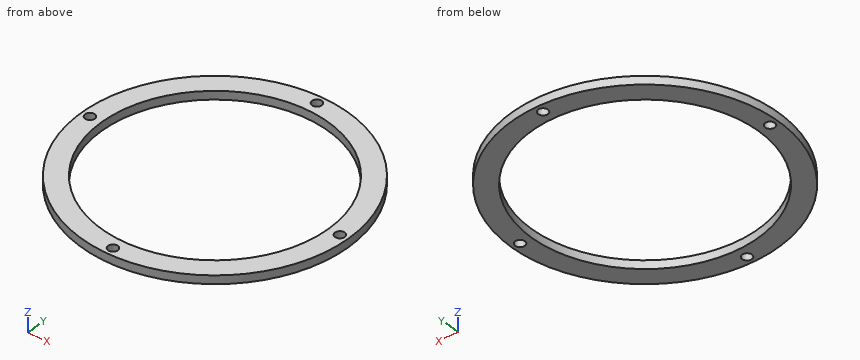
Autodesk Inventor part; units mm, degrees
ref_plane "YZ Plane" through (0, 0, 0) normal (1, 0, 0) x (0, 1, 0)
ref_plane "XZ Plane" through (0, 0, 0) normal (0, 1, 0) x (-1, 0, 0)
ref_plane "XY Plane" through (0, 0, 0) normal (0, 0, 1) x (1, 0, 0)
sketch "Sketch1" plane through (0, 0, 0) normal (0, 0, 1) x (1, 0, 0)
  circle A0 centre (0, 0) radius 48
  circle A1 centre (0, 0) radius 40.75
  line L0 (0, 0) -> (0, 45)
  circle A2 centre (0, 45) radius 1.75
  circle A3 centre (-45, 0) radius 1.75
  circle A4 centre (0, -45) radius 1.75
  circle A5 centre (45, 0) radius 1.75
  dimension "d0" = 96
  dimension "d1" = 81.5
  dimension "d2" = 45
  dimension "d3" = 3.5
  dimension "d6" = 360
extrude "Extrusion1" add sketch "Sketch1" along normal blind 3
properties part number "arm_0_bottom_top_lock"
Geometry check sheet. Reference: the model listing, model coordinates, mm. Give positions to 0.01 mm unless a question says otherwise; leave off trailing zeros. Order: outer loops, then holes, each group sorted by start corner. A loop starts at its lowest first (then second) coordinate and runs counter-clockwise, first axis right, second up.
1) Cross-section at C-C (y = -10). Record the boundary of the cut face in (x, z), then the cut area to 3 significant figures.
Results are:
outline: (-46.95, 0) - (-39.5, 0) - (-39.5, 3) - (-46.95, 3) - close; (39.5, 0) - (46.95, 0) - (46.95, 3) - (39.5, 3) - close
area: 44.7 mm2
2) Cross-section at A-A (y = 0). Record the boundary of the cut face in (x, z), then the cut area to 3 significant figures.
Results are:
outline: (-48, 0) - (-46.75, 0) - (-46.75, 3) - (-48, 3) - close; (-43.25, 0) - (-40.75, 0) - (-40.75, 3) - (-43.25, 3) - close; (40.75, 0) - (43.25, 0) - (43.25, 3) - (40.75, 3) - close; (46.75, 0) - (48, 0) - (48, 3) - (46.75, 3) - close
area: 22.5 mm2
3) Cross-section at D-D (x = -16). Record the boundary of the cut face in (y, z).
Results are:
outline: (-45.25, 0) - (-37.48, 0) - (-37.48, 3) - (-45.25, 3) - close; (37.48, 0) - (45.25, 0) - (45.25, 3) - (37.48, 3) - close
4) Gauge pin test, flat ends, axial feed: pin 1 (1 mm diameter, centred on y = -15, z = 1, fed in from +X); pin 2 (3 mm diameter, centred on x = 0, y = 45, fed in from -Z). Record the tip position at first contact, or that the pin passes through.
Results are:
pin 1: stops at x = 45.76
pin 2: passes through
5) Material ranges on probe 1 along Y at (x, z) = (0, 1.6); probe 2 along X at (y, z) = (-24, 1.7); probe 3 along X at (y, z) = (-12, 1.1), recorded low to high.
Results are:
probe 1: y = -48 to -46.75, -43.25 to -40.75, 40.75 to 43.25, 46.75 to 48
probe 2: x = -41.57 to -32.93, 32.93 to 41.57
probe 3: x = -46.48 to -38.94, 38.94 to 46.48
